Read the model definition and answer for the solid it produces. Units are mm, in the model's axes. A direction names the side the tool comes from. Coordinates: 2 decimals unless noted, no trailing zeros. Write each loop counter-clockwise with the first axis right and the second up, starting at its lowest first coordinate (ties: lowest second). Pieces come first, ordered by that corner, then holes. Notation, with made-up numbers: (-38.5, 42) -> (-11.5, 42) arc R17 ccw to (-11.5, 61) -> close; hole circle Ø3 at (68.25, 55). An arc over 180 degrees is marked (long way). Answer in a Markdown table with one row per item. Add a question column.
Item 1: Section B-B on y = -17.75 is taken. Write down the section's boundary in (x, z) (1 decimal), then the cut area to 3 significant figures.
Item 2: Given pin 1 Ø3 at (x, z) = (15.5, 10.5) entering from +Y; pin 2 Ø1 at (x, z) = (31.5, 4) entering from -Y; pin 3 Ø3 at (y, z) = (-12, 6) entering from -X, each flat-ended and moving along its own axis, determine where each tip first touches the part or whether it passes through.
Item 3: Which of the six approach directions +Z, -Z, +X, -X, +Y, -Y give full straight-line access (tool end or side, diameter ignored) to faces 1 (the face through (19, -19.766, 8)), 2 (the face through (1.143, -12, 8)), 3 (the face through (19, -4.531, 8)), 4 (the face through (36.711, -12, 8))?
Item 4: Straight lines are drawn through the part: line 1 (X direction, y = -9.5, z = 11.25); line 2 (Y direction, x = 5.5, z = 5); line 3 (Z direction, x = 36.5, y = -21.5) (3 decimals). For each, find the intervals that lie inside material, in ascending order. Write a range as from..to.
Item 5: Section D-D on y = -3.75 is taken. Write down the section's boundary in (x, z) (3 decimals), then the cut area to 3 significant figures.
Item 6: Section C-C on z = 8 is taken. Write down the section's boundary in (x, y).
```python
from build123d import *

# Parameters (mm, degrees)
F0_W     = 38.1
F0_H     = 25.4
F1_DEPTH = 3.175
F2_SIZE  = 3.17499
F3_W     = 35.5673587183
F3_H     = 15.2347986586
F4_DEPTH = 9.525


# Not quite as in the source:
# - a fillet or chamfer is up to 0.001 mm smaller than in the source, because OpenCascade refuses the exact size


with BuildPart() as f1:
    # F0 (on Top) → F1 (new body)
    with BuildSketch(Plane.XY):
        with Locations((19.05, -12.7)):
            Rectangle(F0_W, F0_H)
    extrude(amount=F1_DEPTH)

    # F2 (size 3.175 in the source; OpenCascade refuses exactly that, so slightly less here)
    f2_edges = [f1.edges().sort_by_distance(p)[0] for p in [
        (19.05, -25.4, 3.175),
        (19.05, 0, 3.175),
    ]]
    chamfer(f2_edges, length=F2_SIZE)

    # F3 (on face) → F4 (join)
    with BuildSketch(Plane.XY.offset(3.175)):
        with Locations((18.9271715353, -12.1486445423)):
            Rectangle(F3_W, F3_H)
    extrude(amount=F4_DEPTH)


solid = f1.part
```
Results below:
| question | item | result |
|---|---|---|
| 1 | outline | (0, 0) -> (38.1, 0) -> (38.1, 3.2) -> (36.7, 3.2) -> (36.7, 12.7) -> (1.1, 12.7) -> (1.1, 3.2) -> (0, 3.2) -> close |
| 1 | area | 460 mm2 |
| 2 | pin 1 | stops at y = -4.53 |
| 2 | pin 2 | stops at y = -19.77 |
| 2 | pin 3 | stops at x = 1.14 |
| 3 | face 1 | +Z, +X, -X, -Y |
| 3 | face 2 | +Z, -X, +Y, -Y |
| 3 | face 3 | +Z, +X, -X, +Y |
| 3 | face 4 | +Z, +X, +Y, -Y |
| 4 | line 1 | x = 1.14..36.71 |
| 4 | line 2 | y = -19.77..-4.53 |
| 4 | line 3 | z = 0..3.175 |
| 5 | outline | (0, 0) -> (38.1, 0) -> (38.1, 3.175) -> (0, 3.175) -> close |
| 5 | area | 121 mm2 |
| 6 | outline | (1.14, -19.77) -> (36.71, -19.77) -> (36.71, -4.53) -> (1.14, -4.53) -> close |
